Source: CAD feature listing. Evaluate the final solid. Frame: model axes, mm. A direction names the side the tool comes from. Round coordinates to 2 decimals unless told otherwise and drop trailing zeros. Loops run counter-clockwise (first coordinate to the right, second up) from the corner with the lowest first, then second, coordinate; pieces in that order, holes last. Notation, with made-up numbers: (89.5, 23.25) -> (133.5, 23.25) arc R18 ccw to (133.5, 38.25) -> close; hole circle Ø9 at (-20, 86). An arc over 180 degrees is marked (long way). Put each result on its own line as item: value. Start each with the question number.
1. Cut plane A-A (z = -57). Return the cut outline in (x, y).
2. Cut plane B-B (y = 70.5). Return the cut outline in (x, z), then the cut area to 3 significant figures.
3. Cut plane D-D (x = -35). Return the cut outline in (y, z).
4. Cut plane C-C (z = -12.5). Return the cut outline in (x, y).
5. Draft query along Y for faces 1 (the flat face through (94, 63, 0)), 2 (the flat face through (15, 0, -69)), 3 (the flat face through (98, 63, -3)). Return one class per face: pulls with the +Y half, pulls with the -Y half, needs draft (parallel to the pull), parting line crosses it, or undercut.
6. Set-up query: faces 4 (the flat face through (89, 178, -13)), 5 (the flat face through (0, 123, -85)), 6 (the flat face through (6, 5, -71)), 7 (the flat face through (70.9, 63.2, -42.2)), 8 (the flat face through (-98, 63, -3)). Return all of +Z, -Z, +X, -X, +Y, -Y with unobstructed straight access to the full face (end or side cutting, diameter ignored); none if empty.
7. Material intervals for L1, parallel to Y at x = -93.5, z = -13; L2, parallel to X at y = 1, z = -85; L3, parallel to Y at x = -36.5, z = -69.5, sorted ascending.
8. Contact query for flat-ended pins moving along their axis: pin 1 (8 mm diameter, centred on y = 78.5, z = -57.5, fed in from +X); pin 2 (1.5 mm diameter, centred on x = -59.5, y = 105, fed in from +Z); pin 3 (5 mm diameter, centred on x = -6.5, y = 56.5, fed in from +Z). Output: stop coordinate, or through.
```python
from build123d import *

# Parameters (mm, degrees)
BOSS_EXTRUDE1_DEPTH = 5
BOSS_EXTRUDE2_DEPTH = 118
BOSS_EXTRUDE3_DEPTH = 5
BOSS_EXTRUDE4_DEPTH = 50
BOSS_EXTRUDE5_DEPTH = 10
SKETCH6_R           = 2
CUT_EXTRUDE1_DEPTH  = 10
SKETCH7_R           = 2
CUT_EXTRUDE2_DEPTH  = 10


with BuildPart() as part:
    # Sketch1 → Boss-Extrude1 (new body)
    with BuildSketch(Plane(origin=(0, 0, 0), x_dir=(1, 0, 0), z_dir=(0, 1, 0))):
        with BuildLine():
            Line((-103.923048454, 0), (-70, 0))
            ThreePointArc((-70, 0), (0, 70), (70, 0))
            Line((70, 0), (103.923048454, 0))
            Line((103.923048454, 0), (51.961524227, 90))
            Line((51.961524227, 90), (-51.961524227, 90))
            Line((-51.961524227, 90), (-103.923048454, 0))
        make_face()
    extrude(amount=BOSS_EXTRUDE1_DEPTH)

    # Sketch2 → Boss-Extrude2 (add)
    with BuildSketch(Plane(origin=(0, 5, 0), x_dir=(1, 0, 0), z_dir=(0, 1, 0))):
        with BuildLine():
            Line((-95.262794416, 0), (-81, 0))
            ThreePointArc((-81, 0), (0, 81), (81, 0))
            Line((81, 0), (95.262794416, 0))
            Line((95.262794416, 0), (103.923048454, 0))
            Line((103.923048454, 0), (102.190997647, 3))
            Line((102.190997647, 3), (93.530743609, 3))
            Line((93.530743609, 3), (47.631397208, 82.5))
            Line((47.631397208, 82.5), (-47.631397208, 82.5))
            Line((-47.631397208, 82.5), (-93.530743609, 3))
            Line((-93.530743609, 3), (-102.190997647, 3))
            Line((-102.190997647, 3), (-103.923048454, 0))
            Line((-103.923048454, 0), (-95.262794416, 0))
        make_face()
    extrude(amount=BOSS_EXTRUDE2_DEPTH)

    # Sketch3 → Boss-Extrude3 (add)
    with BuildSketch(Plane(origin=(0, 123, 0), x_dir=(1, 0, 0), z_dir=(0, 1, 0))):
        with BuildLine():
            Line((-103.923048454, 0), (-81, 0))
            ThreePointArc((-81, 0), (0, 81), (81, 0))
            Line((81, 0), (103.923048454, 0))
            Line((103.923048454, 0), (51.961524227, 90))
            Line((51.961524227, 90), (-51.961524227, 90))
            Line((-51.961524227, 90), (-103.923048454, 0))
        make_face()
    extrude(amount=BOSS_EXTRUDE3_DEPTH)

    # Sketch4 → Boss-Extrude4 (add)
    with BuildSketch(Plane(origin=(0, 128, 0), x_dir=(1, 0, 0), z_dir=(0, 1, 0))):
        with BuildLine():
            Line((84.870489571, 33), (73.972968036, 33))
            ThreePointArc((73.972968036, 33), (-16.869937598, 79.22376667), (-81, 0))
            Line((-81, 0), (-103.923048454, 0))
            Line((-103.923048454, 0), (-51.961524227, 90))
            Line((-51.961524227, 90), (51.961524227, 90))
            Line((51.961524227, 90), (84.870489571, 33))
        make_face()
    extrude(amount=BOSS_EXTRUDE4_DEPTH)

    # Sketch5 → Boss-Extrude5 (add)
    with BuildSketch(Plane(origin=(0, 178, 0), x_dir=(1, 0, 0), z_dir=(0, 1, 0))):
        with BuildLine():
            Line((-103.923048454, 0), (-51.961524227, 90))
            Line((-51.961524227, 90), (51.961524227, 90))
            Line((51.961524227, 90), (103.923048454, 0))
            Line((103.923048454, 0), (81, 0))
            ThreePointArc((81, 0), (0, 81), (-81, 0))
            Line((-81, 0), (-103.923048454, 0))
        make_face()
    extrude(amount=BOSS_EXTRUDE5_DEPTH)

    # Sketch6 → Cut-Extrude1 (cut)
    with BuildSketch(Plane.XY):
        with Locations((92.461524227, 113)):
            Circle(SKETCH6_R)
        with Locations((92.461524227, 25)):
            Circle(SKETCH6_R)
        with Locations((-92.461524227, 25)):
            Circle(SKETCH6_R)
        with Locations((-92.461524227, 113)):
            Circle(SKETCH6_R)
    extrude(amount=-CUT_EXTRUDE1_DEPTH, mode=Mode.SUBTRACT)

    # Sketch7 → Cut-Extrude2 (cut)
    with BuildSketch(Plane.XZ):
        with Locations(Location((-30, -85, 0), (0, 0, 270))):
            Circle(SKETCH7_R)
        with Locations(Location((30, -85, 0), (0, 0, 270))):
            Circle(SKETCH7_R)
    extrude(amount=-CUT_EXTRUDE2_DEPTH, mode=Mode.SUBTRACT)


solid = part.part
```
Solution:
1. outline: (-71.01, 0) -> (-40.63, 0) -> (-40.63, 5) -> (-57.55, 5) -> (-57.55, 188) -> (-71.01, 188) -> (-71.01, 123) -> (-62.35, 123) -> (-62.35, 5) -> (-71.01, 5) -> close; (40.63, 0) -> (71.01, 0) -> (71.01, 5) -> (62.35, 5) -> (62.35, 123) -> (71.01, 123) -> (71.01, 188) -> (57.55, 188) -> (57.55, 5) -> (40.63, 5) -> close
2. outline: (-103.92, 0) -> (-102.19, -3) -> (-93.53, -3) -> (-47.63, -82.5) -> (47.63, -82.5) -> (93.53, -3) -> (102.19, -3) -> (103.92, 0) -> (81, 0) arc R81 cw to (-81, 0) -> close
2. area: 1,530 mm^2
3. outline: (0, -90) -> (5, -90) -> (5, -82.5) -> (123, -82.5) -> (123, -90) -> (188, -90) -> (188, -73.05) -> (5, -73.05) -> (5, -60.62) -> (0, -60.62) -> close
4. outline: (-96.71, 0) -> (-68.87, 0) -> (-68.87, 5) -> (-80.03, 5) -> (-80.03, 188) -> (-96.71, 188) -> (-96.71, 123) -> (-88.05, 123) -> (-88.05, 5) -> (-96.71, 5) -> close; (68.87, 0) -> (96.71, 0) -> (96.71, 5) -> (88.05, 5) -> (88.05, 123) -> (96.71, 123) -> (96.71, 128) -> (80.03, 128) -> (80.03, 5) -> (68.87, 5) -> close; (80.03, 178) -> (96.71, 178) -> (96.71, 188) -> (80.03, 188) -> close
5. face 1: needs draft
5. face 2: pulls with the -Y half
5. face 3: undercut
6. face 4: +Z, +X
6. face 5: -Z
6. face 6: +Z, +Y
6. face 7: -Z, +X
6. face 8: -Z, -X
7. L1: y = 0 to 5, 123 to 188
7. L2: x = -54.85 to -32, -28 to 28, 32 to 54.85
7. L3: y = 0 to 5
8. pin 1: stops at x = 64.37
8. pin 2: stops at z = -54.14
8. pin 3: stops at z = -80.5
